```python
from build123d import *

# Parameters (mm, degrees)
ESTRUSIONE_ESTRUSIONE1_DEPTH = 5.7


with BuildPart() as part:
    # Model → Estrusione-Estrusione1 (new body)
    with BuildSketch(Plane.XY):
        with BuildLine():
            Line((-5, 0.09), (-5, -3.254122143))
            add(Edge.make_bspline(
                [(-5, -3.254122143), (-122.039878304, -31.264583812), (-115.130671173, 174.542277049), (-11.818324795, 129.448781979)],
                knots=[0, 0, 0, 0, 1, 1, 1, 1], degree=3))
            Line((-11.818324795, 129.448781979), (-19.584652517, 111.22))
            Line((-19.584652517, 111.22), (-40.0225, 111.22))
            Line((-40.0225, 111.22), (-40.0225, 105.61))
            Line((-40.0225, 105.61), (-20.998922906, 105.61))
            Line((-20.998922906, 105.61), (-40.0225, 55.61))
            Line((-40.0225, 55.61), (-55.0225, 55.61))
            Line((-55.0225, 55.61), (-55.0225, 50))
            Line((-55.0225, 50), (-40.0225, 50.008559229))
            Line((-40.0225, 50.008559229), (-11.818324795, 5.7))
            Line((-11.818324795, 5.7), (-25.0225, 5.7))
            Line((-25.0225, 5.7), (-25.0225, 0.09))
            Line((-25.0225, 0.09), (-5, 0.09))
        make_face()
    extrude(amount=ESTRUSIONE_ESTRUSIONE1_DEPTH)


solid = part.part
```
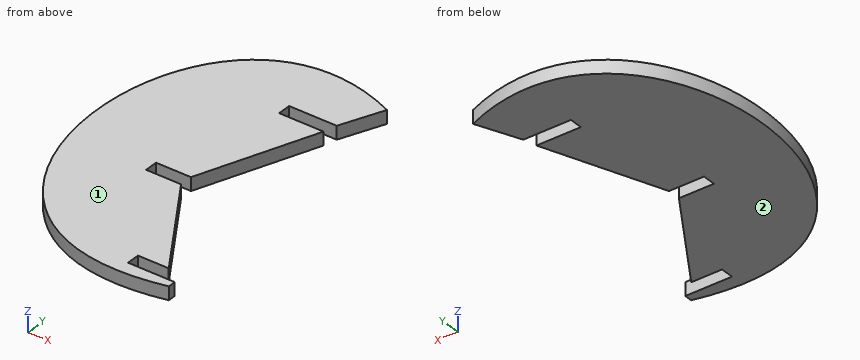
Geometry check sheet. Reference: the model listing, model coordinates, mm. Face numbers are marked on the shaded views. Give positions to 0.01 mm unless a question says otherwise; leave off trailing zeros. Answer in a Markdown table with one row per item. Add a question column.
Q1. Material ranges on probe 1 along Y at (x, z) = (-16, 2.7); probe 2 along Y at (x, z) = (-17.5, 2.75); probe 3 along Y at (x, z) = (-43, 4.25), recorded low to high. Write a range as from..to.
Q2. Gauge pin test, flat ends, axial feed: pin 1 (3 mm diameter, centred on x = -17.5, z = 4, fed in from -Y); pin 2 (3 mm diameter, centred on y = 3, z = 4, fed in from +X); pin 3 (1.5 mm diameter, centred on y = 19.5, z = 1, fed in from +X). Record the tip position at first contact, or that the pin passes through.
Q3. Cross-section at A-A, the plane x = -26.5. Count the separate pieces of the cut face and the enclosed holes in it, then the cut area to 3 significant figures.
Q4. Mould release check, pull along Z, two halves, no side actions. Record for the marked faces 1 and 2: pulls with the +Z half, pulls with the -Z half, needs draft (parallel to the pull), parting line crosses it, or undercut.
Check values:
| question | item | result |
|---|---|---|
| 1 | probe 1 | y = -5.26..0.09, 5.7..12.27, 119.63..131.16 |
| 1 | probe 2 | y = -5.43..0.09, 5.7..14.63, 116.11..131.71 |
| 1 | probe 3 | y = -3.78..50.01, 55.61..135.83 |
| 2 | pin 1 | stops at y = -5.57 |
| 2 | pin 2 | stops at x = -25.02 |
| 2 | pin 3 | stops at x = -20.13 |
| 3 | separate pieces | 3 |
| 3 | enclosed holes | 0 |
| 3 | area | 412 mm^2 |
| 4 | face 1 | pulls with the +Z half |
| 4 | face 2 | pulls with the -Z half |
